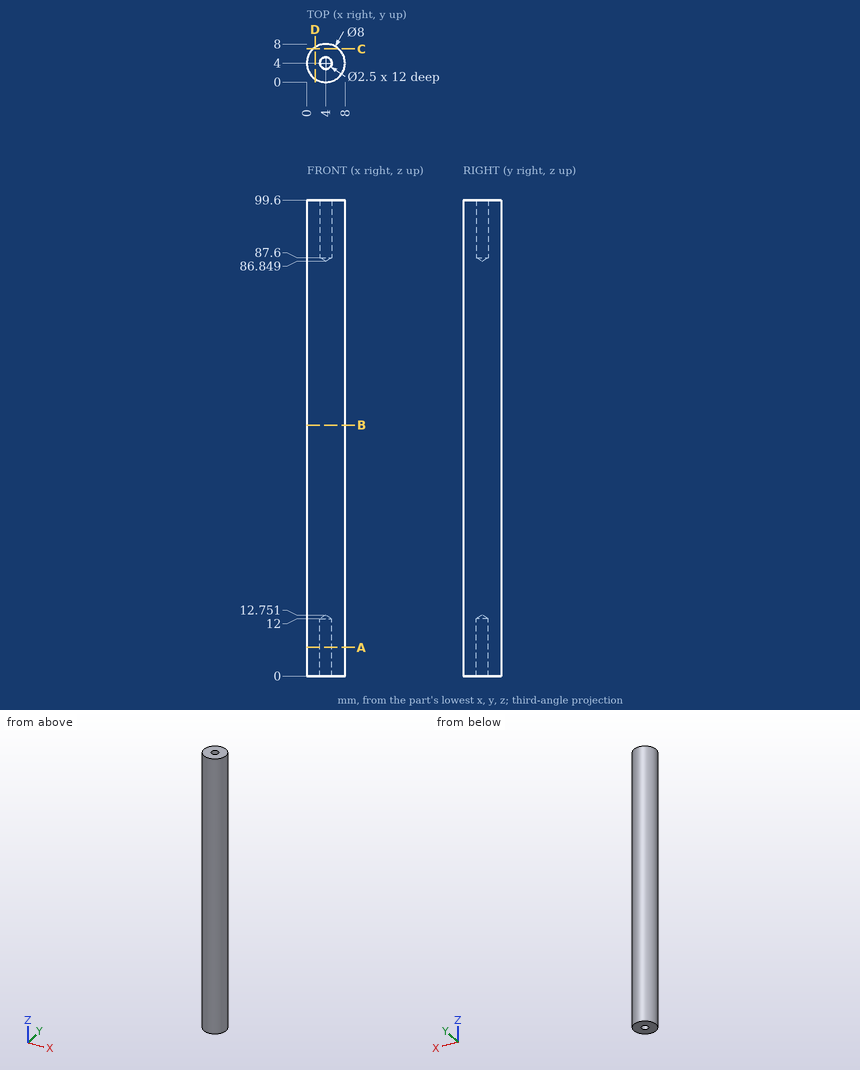
Part print with two shaded views. Sizes in mm from the minimum x, y, z corner. Round coordinates to 2 decimals unless told otherwise and drop trailing zeros. Order: outer loops, then holes, each group sorted by start corner. A loop starts at its lowest first (then second) coordinate and runs counter-clockwise, first axis right, second up. Notation, with made-up numbers: (80, 6.5) - (122, 6.5) arc R30 cw to (122, 28.5) - close; hole circle Ø3 at (78, 18). An arc over 180 degrees is marked (long way). Answer in a Markdown table with one row per item. Add a question column.
(1) Drop flat-ended pins along their axis: pin 1 Ø1.5 at (y, z) = (1, 11.5) entering from +X; pin 2 Ø1.5 at (x, z) = (2, 12) entering from +Y; pin 3 Ø2 at (x, y) = (4, 4) entering from -Z. Give the stop position or say it passes through.
(2) Probe L1, parallel to Y at x = 4, z = 93.5; L2, parallel to X at y = 3.75, z = 78. List the from-to ranges inside material, lowest first. Write a range as [from, to].
(3) Band-saw the part on D-D on x = 1.75. List the corners of the cut face in (y, z).
(4) Band-saw the part on C-C on y = 7. List the corners of the cut face in (x, z).
(5) Band-saw the part on A-A on z = 6. List the corners of the cut face in (x, y), and give its area (3 significant figures).
(6) Band-saw the part on B-B on z = 52.5. List the corners of the cut face in (x, y).
Data:
| question | item | result |
|---|---|---|
| 1 | pin 1 | stops at x = 7.31 |
| 1 | pin 2 | stops at y = 7.8 |
| 1 | pin 3 | stops at z = 12.15 |
| 2 | L1 | y = [0, 2.75], [5.25, 8] |
| 2 | L2 | x = [0.01, 7.99] |
| 3 | outline | (0.69, 0) - (7.31, 0) - (7.31, 99.6) - (0.69, 99.6) - close |
| 4 | outline | (1.35, 0) - (6.65, 0) - (6.65, 99.6) - (1.35, 99.6) - close |
| 5 | outline | circle Ø8 at (4, 4); hole circle Ø2.5 at (4, 4) |
| 5 | area | 45.4 mm^2 |
| 6 | outline | circle Ø8 at (4, 4) |
